Source: CAD feature listing. Evaluate the final solid. Frame: model axes, mm. Face numbers are marked on the shaded views. A direction names the side the tool comes from. Give positions to 0.01 mm unless a question says otherwise; leave off trailing zeros. Order: outer loops, then holes, each group sorted by start corner. A loop starts at its lowest first (then second) coordinate and runs counter-clockwise, first axis right, second up. Notation, with made-up numbers: M 74,-23 L 131,-23 A9 ccw 131,-6 Z; hole C -10,34 d2. An arc over 180 degrees is marked long. Answer in a Markdown table with one row per item. Add a question column.
(1) Set-up query: the marked faces 1, 2 and 3. Return all of +Z, -Z, +X, -X, +Y, -Y with unobstructed straight access to the full face (end or side cutting, diameter ignored); none if empty.
(2) Pin query (flat end, axial travel): P1, Ø3, axis at y = -36.5, z = 19, coming from the +X side; P2, Ø5, axis at x = 40.5, z = 24, coming from the -Y side; P3, Ø10, axis at x = 19, z = 11, coming from the -Y side; P4, Ø22.5, axis at x = 0, y = -12.7, coming from the +Z side. Return the tip coordinate at first contact, or that it passes through.
(3) Mould query, pull axis Y, two halves, no side actions, for the marked faces 4, 5 and 6. Classes: pulls with the +Y half, pulls with the -Y half, needs draft (parallel to the pull), parting line crosses it, or undercut.
(4) Section query B-B, the plane y = 0. Return loops of the section in (x, z) (3 decimals), plus the area to 3 significant figures.
(5) Material intervals for line 1 along Y through (x, z) = (0, 40.5); line 2 along Y through (x, z) = (0, 25); line 3 along X through (y, z) = (-0.5, 6), sorted ascending.
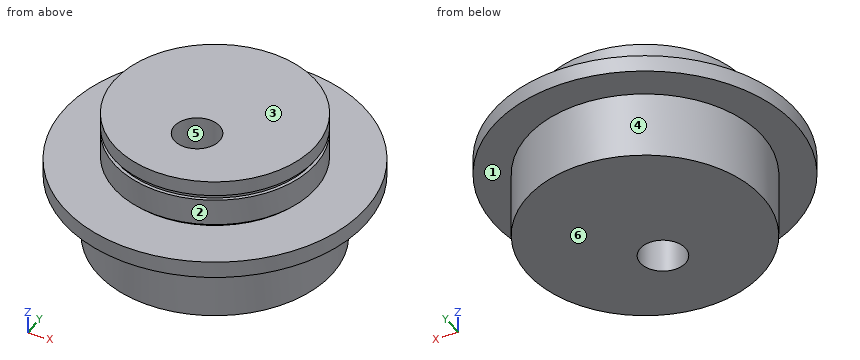
from build123d import *

# Parameters (mm, degrees)
SKETCH1_R               = 44.45
BOSS_EXTRUDE1_DEPTH     = 25.4
SKETCH2_R               = 36.83
BOSS_EXTRUDE2_DEPTH     = 25.4
SKETCH7_R               = 38.1
BOSS_EXTRUDE3_DEPTH     = 5.715
BOSS_EXTRUDE4_START     = -5.715
SKETCH8_R               = 38.1
BOSS_EXTRUDE4_DEPTH     = 5.715
BOSS_EXTRUDE6_START     = 7.62
SKETCH11_R              = 38.1
BOSS_EXTRUDE6_DEPTH     = 10.16
SKETCH12_R              = 57.15
BOSS_EXTRUDE7_DEPTH     = 6.35
CUT_EXTRUDE1_DEPTH      = 96.461432003
CUT_EXTRUDE1_DEPTH_BACK = 96.461432003
SKETCH3_R               = 8.5725


with BuildPart() as part:
    # Sketch1 → Boss-Extrude1 (new body)
    with BuildSketch(Plane.XY):
        Circle(SKETCH1_R)
    extrude(amount=BOSS_EXTRUDE1_DEPTH)

    # Sketch2 → Boss-Extrude2 (add)
    with BuildSketch(Plane.XY.offset(25.4)):
        Circle(SKETCH2_R)
    extrude(amount=BOSS_EXTRUDE2_DEPTH)

    # Sketch7 → Boss-Extrude3 (add)
    with BuildSketch(Plane.XY.offset(25.4)):
        Circle(SKETCH7_R)
    extrude(amount=BOSS_EXTRUDE3_DEPTH)

    # Sketch8 → Boss-Extrude4 (add)
    with BuildSketch(Plane.XY.offset(50.8).offset(BOSS_EXTRUDE4_START)):
        Circle(SKETCH8_R)
    extrude(amount=BOSS_EXTRUDE4_DEPTH)

    # Sketch11 → Boss-Extrude6 (add)
    with BuildSketch(Plane.XY.offset(25.4).offset(BOSS_EXTRUDE6_START)):
        Circle(SKETCH11_R)
    extrude(amount=BOSS_EXTRUDE6_DEPTH)

    # Sketch12 → Boss-Extrude7 (add)
    with BuildSketch(Plane.XY.offset(25.4)):
        Circle(SKETCH12_R)
    extrude(amount=BOSS_EXTRUDE7_DEPTH)

    # Sketch3 → Cut-Extrude1 (cut, two sides: drawn at the far end of the back side and taken through both)
    with BuildSketch(Plane.XY.offset(50.8).offset(-CUT_EXTRUDE1_DEPTH_BACK)):
        with Locations((0, -12.7)):
            Circle(SKETCH3_R)
    extrude(amount=CUT_EXTRUDE1_DEPTH + CUT_EXTRUDE1_DEPTH_BACK, mode=Mode.SUBTRACT)


solid = part.part
Values follow:
| question | item | result |
|---|---|---|
| 1 | face 1 | -Z |
| 1 | face 2 | +Z |
| 1 | face 3 | +Z, +X, -X, +Y, -Y |
| 2 | P1 | stops at x = 27.4 |
| 2 | P2 | stops at y = -42.3 |
| 2 | P3 | stops at y = -42.19 |
| 2 | P4 | stops at z = 50.8 |
| 3 | face 4 | parting line crosses it |
| 3 | face 5 | undercut |
| 3 | face 6 | needs draft |
| 4 | outline | M -57.15,25.4 L -44.45,25.4 L -44.45,0 L 44.45,0 L 44.45,25.4 L 57.15,25.4 L 57.15,31.75 L 36.83,31.75 L 36.83,33.02 L 38.1,33.02 L 38.1,43.18 L 36.83,43.18 L 36.83,45.085 L 38.1,45.085 L 38.1,50.8 L -38.1,50.8 L -38.1,45.085 L -36.83,45.085 L -36.83,43.18 L -38.1,43.18 L -38.1,33.02 L -36.83,33.02 L -36.83,31.75 L -57.15,31.75 Z |
| 4 | area | 4,430 mm² |
| 5 | line 1 | y = -38.1 to -21.27, -4.13 to 38.1 |
| 5 | line 2 | y = -44.45 to -21.27, -4.13 to 44.45 |
| 5 | line 3 | x = -44.45 to 44.45 |
